Autodesk Inventor part; units mm, degrees
ref_plane "YZ Plane" through (0, 0, 0) normal (1, 0, 0) x (0, 1, 0)
ref_plane "XZ Plane" through (0, 0, 0) normal (0, 1, 0) x (-1, 0, 0)
ref_plane "XY Plane" through (0, 0, 0) normal (0, 0, 1) x (1, 0, 0)
sketch "Sketch3" plane through (0, 0, 0) normal (0, 1, 0) x (-1, 0, 0)
  circle A0 centre (0, 0) radius 39.5
  line L0 (0, 0) -> (-150, 0)
  line L1 (-150, 0) -> (-150, 25)
  line L2 (-150, 0) -> (-150, -25)
  line L3 (-150, 0) -> (-150, 1.869)
  line L4 (-150, 0) -> (32.5266, 22.4114) construction
  line L5 (-150, 0) -> (33.8973, 0) construction
  arc A1 (-61.0323, 2.8576) -> (32.5266, 22.4114) centre (-62.3689, 242.8539) ccw
  arc A2 (32.5266, -22.4114) -> (-61.0323, -2.8576) centre (-62.3689, -242.8539) ccw
  circle A3 centre (0, 0) radius 5
  line L6 (-150, 0.9345) -> (-100.7064, 2)
  line L7 (-150, -0.9345) -> (-61.0323, -2.8576)
  line L8 (-150, 0.9345) -> (-61.0323, 2.8576)
  point P0 (-150, -1.869)
  point P1 (-150, -6)
  point P2 (32.5266, -22.4114)
  point P3 (-100.7064, -2)
  point P4 (-39.3005, 3.9651)
  point P5 (-39.3005, -3.9651)
  point P6 (-150, 0.9345)
  dimension "d17" = 79
  dimension "d18" = 150
  dimension "d19" = 25
  dimension "d20" = 25
  dimension "d22" = 7
  dimension "d23" = 10
  dimension "d26" = 240
  dimension "d27" = 1.238
  dimension "d28" = 25.6262
  dimension "d29" = 50.7411
  dimension "d30" = 2
  dimension "d33" = 1.238
extrude "Extrusion2" add sketch "Sketch3" along normal blind 25 contours A0 A2 A1 | A0 L0 L1 L6 L8 A1 | A2 L7 L2 L0 A0
sketch "Sketch4" plane through (0, 25, 0) normal (0, 1, 0) x (1, 0, 0)
  arc A0 (-28.2743, -20.6292) -> (-28.2743, 20.6292) centre (0, 0) ccw construction
  arc A1 (61.0323, -2.8576) -> (-32.5266, -22.4114) centre (62.3689, -242.8539) ccw
  arc A2 (-32.5266, 22.4114) -> (61.0323, 2.8576) centre (62.3689, 242.8539) ccw
  arc A3 (-28.2743, 20.6292) -> (-28.2743, -20.6292) centre (0, 0) ccw
  arc A4 (-32.5266, 22.4114) -> (-32.5266, -22.4114) centre (0, 0) ccw
  dimension "d35" = 70
extrude "Extrusion3" cut sketch "Sketch4" against normal through all
sketch "Sketch5" plane through (0, 25, 0) normal (0, 1, 0) x (1, 0, 0)
  circle A0 centre (0, 0) radius 5
  line L0 (-3, 1) -> (-7, 1)
  line L1 (-7, 1) -> (-7, -1)
  line L2 (-7, -1) -> (-3, -1)
  line L3 (-3, -1) -> (-3, 1)
  line L4 (-3, 1) -> (-7, -1) construction
  line L5 (-7, 1) -> (-3, -1) construction
  point P0 (-5, 0)
  point P1 (-4.899, -1)
  point P2 (-4.899, 1)
  dimension "d42" = 5
  dimension "d43" = 2
  dimension "d44" = 4
  dimension "d45" = 3
sketch "Sketch6" plane through (0, 25, 0) normal (0, 1, 0) x (1, 0, 0)
  arc A0 (-5, 0) -> (-5, 0) centre (0, 0) ccw
  line L0 (-7, 1) -> (-5, 1)
  line L1 (-5, -1) -> (-7, -1)
  line L2 (-7, -1) -> (-7, 1)
extrude "Extrusion5" add sketch "Sketch5" against normal blind 25 contours L0 L3 L2 A0 picked at (-3.6629, -0.1118)
sketch "Sketch8" plane through (0, 25, 0) normal (0, 1, 0) x (1, 0, 0)
  line L0 (0, 0) -> (5, 0) construction
  arc A0 (-4.899, -1) -> (-4.899, 1) centre (0, 0) ccw
sketch "Sketch9" plane through (0, 25, 0) normal (0, 1, 0) x (1, 0, 0)
  arc A0 (-28.2743, 20.6292) -> (-28.2743, -20.6292) centre (0, 0) ccw
  arc A1 (-28.2743, 20.6292) -> (61.0323, 2.8576) centre (62.3689, 242.8539) ccw
  arc A2 (61.0323, -2.8576) -> (-28.2743, -20.6292) centre (62.3689, -242.8539) ccw
  line L0 (0, 0) -> (-20, 0) construction
  circle A3 centre (-20, 0) radius 10
  line L1 (0, 0) -> (20, 0) construction
  circle A4 centre (20, 0) radius 5
  line L2 (20, 0) -> (35, 0) construction
  circle A5 centre (35, 0) radius 2.5
  line L3 (35, 0) -> (45, 0) construction
  circle A6 centre (45, 0) radius 1.25
  line L4 (45, 0) -> (55, 0) construction
  circle A7 centre (55, 0) radius 1.25
  line L5 (55, 0) -> (65, 0) construction
  circle A8 centre (65, 0) radius 1.25
  dimension "d50" = 20
  dimension "d51" = 20
  dimension "d52" = 20
  dimension "d53" = 10
  dimension "d54" = 15
  dimension "d55" = 5
  dimension "d60" = 10
  dimension "d61" = 2.5
  dimension "d62" = 10
  dimension "d63" = 2.5
  dimension "d64" = 10
  dimension "d65" = 2.5
extrude "Extrusion6" cut sketch "Sketch9" against normal through all
properties part number "mover_3DPrint"
Design review of the part built by this model. Coordinates are the model's own, in mm. Give positions to 0.01 mm unless a question says otherwise; leave off trailing zeros. Order: outer loops, then holes, each group sorted by start corner. A loop starts at its lowest first (then second) coordinate and runs counter-clockwise, first axis right, second up. Notation, with made-up numbers: (6.25, -14.5) - (43.25, -14.5) arc R5 ccw to (43.25, -6.5) - close; hole circle Ø4 at (-9, 72.5). An arc over 180 degrees is marked (long way). Use a Markdown table: item, result. Add a question column.
(1) Add section B-B on y = 9.5. Give the boundary of the cut face in (x, z), then the cut area to 3 significant figures.
(2) Mouldability with a two-part tool opening along Z and no side actions: class faces 1 (the face through (14.9, 12.325, 7.595)), 2 (the face through (-35, 13, 0)), 3 (the face through (37.31, 12.68, 0.96)) as +Z half, -Z half, draft (parallel to the pull), parting line (faces both ways), or undercut.
(3) Add section D-D on x = 85. Give the boundary of the cut face in (y, z).
(4) Add section C-C on x = 0. Give the boundary of the cut face in (y, z).
(5) Wall thickness on probe 1 along Z at (x, y) = (-20, 19.75); probe 2 along Z at (x, y) = (100.5, 12); probe 3 along Z at (x, y) = (55, 6.75): over which ranges is each line inside the solid? List them lowest first. Write a range as [from, to].
(6) Clearance check with flat-ended pins moving along their axes: P1, Ø3, axis at y = 8.5, z = -15, coming from the -X side; P2, Ø3, axis at x = 35, z = 0, coming from the +Y side; P3, Ø3, axis at x = 26.5, y = 4.5, coming from the +Z side; P4, Ø2, axis at x = -4.5, y = 8, coming from the +Z side. State where each tip first meets the part, or that it passes through.
(7) Add section A-A on x = -20. Give the boundary of the cut face in (y, z), then the cut area to 3 significant figures.
Report:
| question | item | result |
|---|---|---|
| 1 | outline | (-28.27, -20.63) arc R240 cw to (61.03, -2.86) - (150, -0.93) - (150, 0.93) - (100.71, 2) - (61.03, 2.86) arc R240 cw to (-28.27, 20.63) arc R35 ccw to start; hole circle Ø20 at (-20, 0); hole (-4.9, -1) arc R5 ccw (long way) to (-4.9, 1) - (-3, 1) - (-3, -1) - close; hole circle Ø10 at (20, 0); hole circle Ø5 at (35, 0); hole circle Ø2.5 at (45, 0); hole circle Ø2.5 at (55, 0); hole circle Ø2.5 at (65, 0) |
| 1 | area | 1,590 mm² |
| 2 | face 1 | +Z half |
| 2 | face 2 | parting line |
| 2 | face 3 | undercut |
| 3 | outline | (0, -2.34) - (25, -2.34) - (25, 2.34) - (0, 2.34) - close |
| 4 | outline | (0, -11.1) - (25, -11.1) - (25, -5) - (0, -5) - close; (0, 5) - (25, 5) - (25, 11.1) - (0, 11.1) - close |
| 5 | probe 1 | z = [-17.43, -10], [10, 17.43] |
| 5 | probe 2 | z = [-2, 2] |
| 5 | probe 3 | z = [-2.97, -1.25], [1.25, 2.97] |
| 6 | P1 | stops at x = -32.29 |
| 6 | P2 | passes through |
| 6 | P3 | stops at z = 5.78 |
| 6 | P4 | stops at z = 12.65 |
| 7 | outline | (0, -17.43) - (25, -17.43) - (25, -10) - (0, -10) - close; (0, 10) - (25, 10) - (25, 17.43) - (0, 17.43) - close |
| 7 | area | 372 mm² |
